Work out the finished part from the listing and answer in its coordinate system (mm). Face numbers are marked on the shaded views. Round coordinates to 2 decimals unless told otherwise and drop trailing zeros. Write each loop counter-clockwise with the first axis right and the second up, starting at its lowest first coordinate (ties: lowest second). Pieces come first, ordered by that corner, then holes.
1. Determine the mould class of the marked faces 1 and 2 for opening direction Y: pulls with the +Y half, pulls with the -Y half, needs draft (parallel to the pull), parting line crosses it, or undercut.
2. Find section A-A (y = 63.5). Write down the section's boundary in (x, z) (1 decimal).
3. Straight lines are drawn through the part: probe 1 along Y at (x, z) = (-0.5, 194); probe 2 along Y at (x, z) = (0, 111); probe 3 along Z at (x, y) = (0.25, 36.5). For each, find the intervals that lie inside material, in ascending order.
4. Find section B-B (z = 194.5). Write down the section's boundary in (x, y).
5. Flat-ended cylindrical pins translate along their axes: pin 1 Ø4 at (x, z) = (-3.5, 119.5) entering from -Y; pin 2 Ø7 at (x, y) = (0, 0) entering from -Z; pin 3 Ø1.5 at (x, z) = (-5, 134.5) entering from -Y. Find the tip coordinate at first contact, or state that the pin passes through.
```python
from build123d import *

# Parameters (mm, degrees)
SKETCH1_R                = 4.98475
SKETCH1_R_2              = 4.0005
BOSS_EXTRUDE1_DEPTH      = 242.57
BOSS_EXTRUDE2_START      = -39.37
SKETCH2_R                = 6.8326
SKETCH2_R_2              = 4.98475
BOSS_EXTRUDE2_DEPTH      = 39.37
BOSS_EXTRUDE3_DEPTH      = 22.86
BOSS_EXTRUDE3_DEPTH_BACK = 6.35
SKETCH4_R                = 9.7155
SKETCH5_R                = 7.747
CUT_EXTRUDE1_DEPTH       = 22.86
FILLET1_R                = 5.08
BOSS_EXTRUDE5_DEPTH      = 124.46
BOSS_EXTRUDE5_DEPTH_BACK = 15.24
SKETCH6_R                = 7.747
SKETCH6_R_2              = 6.9215
SKETCH7_R                = 9.779
BOSS_EXTRUDE6_DEPTH      = 10.16
CUT_EXTRUDE2_DEPTH       = 217.718250934


with BuildPart() as part:
    # Sketch1 → Boss-Extrude1 (new body)
    with BuildSketch(Plane.XY):
        Circle(SKETCH1_R)
        Circle(SKETCH1_R_2, mode=Mode.SUBTRACT)
    extrude(amount=BOSS_EXTRUDE1_DEPTH)

    # Sketch2 → Boss-Extrude2 (add)
    with BuildSketch(Plane.XY.offset(140.97).offset(BOSS_EXTRUDE2_START)):
        Circle(SKETCH2_R)
        Circle(SKETCH2_R_2, mode=Mode.SUBTRACT)
    extrude(amount=BOSS_EXTRUDE2_DEPTH)

    # Sketch4 → Boss-Extrude3 (add, two sides: drawn at the far end of the back side and taken through both)
    with BuildSketch(Plane(origin=(0, 6.8326, 0), x_dir=(1, 0, 0), z_dir=(0, 1, 0)).offset(-BOSS_EXTRUDE3_DEPTH_BACK)):
        with Locations(Location((0, -121.285, 0), (0, 0, 270))):
            Circle(SKETCH4_R)
    extrude(amount=BOSS_EXTRUDE3_DEPTH + BOSS_EXTRUDE3_DEPTH_BACK)

    # Sketch5 → Cut-Extrude1 (cut)
    with BuildSketch(Plane(origin=(0, 29.6926, 0), x_dir=(1, 0, 0), z_dir=(0, 1, 0))):
        with Locations(Location((0, -121.285, 0), (0, 0, 270))):
            Circle(SKETCH5_R)
    extrude(amount=-CUT_EXTRUDE1_DEPTH, mode=Mode.SUBTRACT)

    # Fillet1
    # the kernel refuses this fillet: 5.08 mm, written as the material it adds along each edge
    # the kernel refuses this fillet: 5.08 mm, written as the material it takes off along each edge
    with BuildSketch(Plane(origin=(0, 0.4826, 121.285), x_dir=(-0.9876010870599544, 0, -0.1569843713176455), z_dir=(0.1569843713176455, 0, -0.9876010870599544))) as fillet1_2_piece_1_section:
        with BuildLine():
            CenterArc((9.7155 - FILLET1_R, FILLET1_R), FILLET1_R, 270, 90)
            Line((9.7155 - FILLET1_R, 0), (9.7155, 0))
            Line((9.7155, 0), (9.7155, FILLET1_R))
        make_face()
    fillet1_2_piece_1 = revolve(axis=Axis((0, 0.4826, 121.285), (0, 1, 0)), revolution_arc=198.063802919, mode=Mode.PRIVATE)
    fillet1_2_piece_1 = fillet1_2_piece_1 - Plane(origin=(0, 0, 123.780869726), x_dir=(1, 0, 0), z_dir=(0, 0, -1)) * Cylinder(6.8326, 39, mode=Mode.PRIVATE)
    add(fillet1_2_piece_1, mode=Mode.SUBTRACT)
    with BuildSketch(Plane(origin=(0, 0.4826, 121.285), x_dir=(0.9876010870599545, 0, 0.15698437131764403), z_dir=(-0.15698437131764403, 0, 0.9876010870599545))) as fillet1_2_piece_2_section:
        with BuildLine():
            CenterArc((9.7155 - FILLET1_R, FILLET1_R), FILLET1_R, 270, 90)
            Line((9.7155, FILLET1_R), (9.7155, 0))
            Line((9.7155, 0), (9.7155 - FILLET1_R, 0))
        make_face()
    fillet1_2_piece_2 = revolve(axis=Axis((0, 0.4826, 121.285), (0, 1, 0)), revolution_arc=198.063802919, mode=Mode.PRIVATE)
    fillet1_2_piece_2 = fillet1_2_piece_2 - Plane(origin=(0, 0, 118.789130045), x_dir=(1, 0, 0), z_dir=(0, 0, -1)) * Cylinder(6.8326, 39, mode=Mode.PRIVATE)
    add(fillet1_2_piece_2, mode=Mode.SUBTRACT)
    with BuildSketch(Plane(origin=(0, 0.4826, 121.285), x_dir=(-0.505713651379917, 0, 0.8627013984038694), z_dir=(-0.8627013984038694, 0, -0.505713651379917))) as fillet1_2_piece_3_section:
        with BuildLine():
            CenterArc((9.7155 - FILLET1_R, FILLET1_R), FILLET1_R, 270, 90)
            Line((9.7155 - FILLET1_R, 0), (9.7155, 0))
            Line((9.7155, 0), (9.7155, FILLET1_R))
        make_face()
    fillet1_2_piece_3 = revolve(axis=Axis((0, 0.4826, 121.285), (0, 1, 0)), revolution_arc=240.757475194, mode=Mode.PRIVATE)
    fillet1_2_piece_3 = fillet1_2_piece_3 - Plane(origin=(0, 0, 129.754845305), x_dir=(1, 0, 0), z_dir=(0, 0, -1)) * Cylinder(6.8326, 39, mode=Mode.PRIVATE)
    add(fillet1_2_piece_3, mode=Mode.SUBTRACT)
    with BuildSketch(Plane(origin=(0, 0.4826, 121.285), x_dir=(0.5057136513799171, 0, -0.8627013984038694), z_dir=(0.8627013984038694, 0, 0.5057136513799171))) as fillet1_2_piece_4_section:
        with BuildLine():
            CenterArc((9.7155 - FILLET1_R, FILLET1_R), FILLET1_R, 270, 90)
            Line((9.7155 - FILLET1_R, 0), (9.7155, 0))
            Line((9.7155, 0), (9.7155, FILLET1_R))
        make_face()
    fillet1_2_piece_4 = revolve(axis=Axis((0, 0.4826, 121.285), (0, 1, 0)), revolution_arc=240.757475194, mode=Mode.PRIVATE)
    fillet1_2_piece_4 = fillet1_2_piece_4 - Plane(origin=(0, 0, 112.815156077), x_dir=(1, 0, 0), z_dir=(0, 0, -1)) * Cylinder(6.8326, 39, mode=Mode.PRIVATE)
    add(fillet1_2_piece_4, mode=Mode.SUBTRACT)

    # Sketch6 → Boss-Extrude5 (add, two sides: drawn at the far end of the back side and taken through both)
    with BuildSketch(Plane(origin=(0, 29.6926, 0), x_dir=(1, 0, 0), z_dir=(0, 1, 0)).offset(-BOSS_EXTRUDE5_DEPTH_BACK)):
        with Locations(Location((0, -121.285, 0), (0, 0, 270))):
            Circle(SKETCH6_R)
        with Locations(Location((0, -121.285, 0), (0, 0, 270))):
            Circle(SKETCH6_R_2, mode=Mode.SUBTRACT)
    extrude(amount=BOSS_EXTRUDE5_DEPTH + BOSS_EXTRUDE5_DEPTH_BACK)

    # Sketch7 → Boss-Extrude6 (add)
    with BuildSketch(Plane(origin=(0, 154.1526, 0), x_dir=(1, 0, 0), z_dir=(0, 1, 0))):
        with Locations(Location((0, -121.285, 0), (0, 0, 270))):
            Circle(SKETCH7_R)
    extrude(amount=BOSS_EXTRUDE6_DEPTH)

    # Sketch8 → Cut-Extrude2 (cut, through all)
    with BuildSketch(Plane(origin=(0, 0, 101.6), x_dir=(-1, 0, 0), z_dir=(0, 0, -1))):
        Polygon((9.779, 164.3126), (-9.779, 164.3126), (9.779, 159.2326), align=None)
    extrude(amount=-CUT_EXTRUDE2_DEPTH, mode=Mode.SUBTRACT)


solid = part.part
```
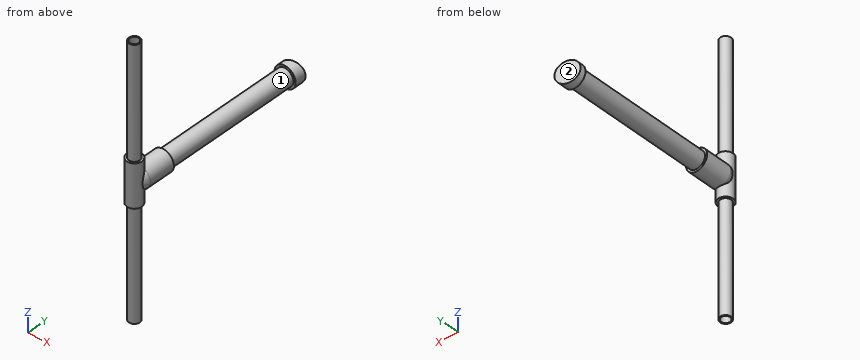
Worked answers:
1. face 1: undercut
1. face 2: pulls with the +Y half
2. outline: circle Ø15.5 at (0, 121.3); hole circle Ø13.8 at (0, 121.3)
3. probe 1: y = -4.96 to -3.97, 3.97 to 4.96
3. probe 2: y = -6.83 to -4, 4 to 6.83
3. probe 3: z = 113.54 to 114.37, 128.2 to 129.03
4. outline: circle Ø9.97 at (0, 0); hole circle Ø8 at (0, 0)
5. pin 1: stops at y = -6.67
5. pin 2: stops at z = 111.57
5. pin 3: stops at y = -5.35
